Can you work these out from the model? Positions are in its coordinate system, mm. Face numbers are marked on the shaded views. A direction names the side the tool comes from. Round coordinates to 2 decimals unless told otherwise and drop trailing zeros. Loops run counter-clockwise (first coordinate to the right, second up) from the corner with the lowest first, then second, coordinate; pieces in that order, holes last. Notation, with made-up numbers: (13, 51.5) -> (54, 51.5) arc R30 ccw to (54, 79.5) -> close; hole circle Ø5 at (45, -1). An arc over 180 degrees is marked (long way). Use a Markdown table: item, result.
from build123d import *

# Parameters (mm, degrees)
BOSS_EXTRU_1_DEPTH = 75
SKETCH3_R          = 30
CUT_EXTRUDE3_DEPTH = 10
ESQUISSE2_R        = 45
BOSS_EXTRU_2_DEPTH = 8
CHANFREIN1_SIZE    = 5
BOSS_EXTRU_3_START = 8
ESQUISSE3_R        = 45
BOSS_EXTRU_3_DEPTH = 8
CHANFREIN2_SIZE    = 5
D_POUILLE5_ANGLE   = 45
D_POUILLE6_ANGLE   = 45
CHANFREIN4_SIZE    = 10
SKETCH2_R          = 45
CUT_EXTRUDE2_DEPTH = 55
FILLET1_R          = 5
CHAMFER1_SIZE      = 8


with BuildPart() as part:
    # Esquisse1 → Boss.-Extru.1 (new body)
    with BuildSketch(Plane.XY):
        with BuildLine():
            Line((95, -48), (95, 48))
            Line((95, 48), (-50, 48))
            Line((-50, 48), (-50, 42))
            Line((-50, 42), (-233.844505579, 42))
            ThreePointArc((-233.844505579, 42), (-295, 0), (-233.844505579, -42))
            Line((-233.844505579, -42), (-50, -42))
            Line((-50, -42), (-50, -48))
            Line((-50, -48), (95, -48))
        make_face()
    extrude(amount=BOSS_EXTRU_1_DEPTH)

    # Sketch3 → Cut-Extrude3 (cut)
    with BuildSketch(Plane.XY.offset(75)):
        Circle(SKETCH3_R)
    extrude(amount=-CUT_EXTRUDE3_DEPTH, mode=Mode.SUBTRACT)

    # Esquisse2 → Boss.-Extru.2 (add)
    with BuildSketch(Plane.XY.offset(75)):
        with Locations(Location((-250, 0, 0), (0, 0, 68.960530219))):
            Circle(ESQUISSE2_R)
    extrude(amount=BOSS_EXTRU_2_DEPTH)

    # Chanfrein1
    chanfrein1_edges = [part.edges().sort_by_distance(p)[0] for p in [
        (-266.155494421, -42, 83),
    ]]
    chamfer(chanfrein1_edges, length=CHANFREIN1_SIZE)

    # Esquisse3 → Boss.-Extru.3 (add)
    with BuildSketch(Plane(origin=(0, 0, 0), x_dir=(-1, 0, 0), z_dir=(0, 0, -1)).offset(BOSS_EXTRU_3_START)):
        with Locations((250, 0)):
            Circle(ESQUISSE3_R)
    extrude(amount=-BOSS_EXTRU_3_DEPTH)

    # Chanfrein2
    chanfrein2_edges = [part.edges().sort_by_distance(p)[0] for p in [
        (-205, 0, -8),
    ]]
    chamfer(chanfrein2_edges, length=CHANFREIN2_SIZE)

    # Dépouille5
    d_pouille5_faces = [part.faces().sort_by_distance(p)[0] for p in [
        (-50, 45, 37.5),
    ]]
    draft(d_pouille5_faces, Plane(origin=(-50, 42, 75), x_dir=(1, 0, 0), z_dir=(0, 1, 0)), D_POUILLE5_ANGLE)

    # Dépouille6
    d_pouille6_faces = [part.faces().sort_by_distance(p)[0] for p in [
        (-50, -45, 37.5),
    ]]
    draft(d_pouille6_faces, Plane(origin=(-50, -42, 75), x_dir=(-1, 0, 0), z_dir=(0, -1, 0)), D_POUILLE6_ANGLE)

    # Chanfrein4
    # the kernel refuses this chamfer: 10 mm, written as the material it takes off along each edge
    with BuildSketch(Plane(origin=(-259.561335458, -42, 75), x_dir=(0, -0.027495876610586317, -0.9996219169112968), z_dir=(1, 0, 0))) as chanfrein4_piece_1_section:
        Polygon((CHANFREIN4_SIZE * 0.999621916911, CHANFREIN4_SIZE * 0.0274958766106), (-CHANFREIN4_SIZE * 0.0274958766106, CHANFREIN4_SIZE * 0.999621916911), (0, 0), align=None)
    chanfrein4_piece_1 = extrude(amount=235.278165338, mode=Mode.PRIVATE)
    chanfrein4_piece_1 = chanfrein4_piece_1 - Plane(origin=(-250, 0, 71.650306889), x_dir=(0.35901098714230106, 0.9333333333333331, 0), z_dir=(0, 0, -1)) * Cylinder(45, 511, mode=Mode.PRIVATE)
    chanfrein4_piece_1 = split(chanfrein4_piece_1, bisect_by=Plane(origin=(-96.832103128, 4.832103128, 71.650306889), z_dir=(-0.7071067811865462, -0.7071067811865488, 0)), keep=Keep.TOP, mode=Mode.PRIVATE)
    add(chanfrein4_piece_1, mode=Mode.SUBTRACT)
    with BuildSketch(Plane(origin=(-259.561335458, -42, 0), x_dir=(0, 0.9996219169112968, -0.027495876610586372), z_dir=(1, 0, 0))) as chanfrein4_piece_2_section:
        Polygon((CHANFREIN4_SIZE * 0.999621916911, CHANFREIN4_SIZE * 0.0274958766106), (-CHANFREIN4_SIZE * 0.0274958766106, CHANFREIN4_SIZE * 0.999621916911), (0, 0), align=None)
    chanfrein4_piece_2 = extrude(amount=235.278165338, mode=Mode.PRIVATE)
    chanfrein4_piece_2 = chanfrein4_piece_2 - Plane(origin=(-250, 0, 3.349693111), x_dir=(-1, 0, 0), z_dir=(0, 0, -1)) * Cylinder(45, 511, mode=Mode.PRIVATE)
    chanfrein4_piece_2 = split(chanfrein4_piece_2, bisect_by=Plane(origin=(-96.832103062, 4.832103062, 3.349693111), z_dir=(-0.7071067811865462, -0.7071067811865488, 0)), keep=Keep.TOP, mode=Mode.PRIVATE)
    add(chanfrein4_piece_2, mode=Mode.SUBTRACT)
    with BuildSketch(Plane(origin=(-24.28317012, 42, 0), x_dir=(0, -0.9996219169112968, -0.027495876610586372), z_dir=(-1, 0, 0))) as chanfrein4_piece_3_section:
        Polygon((CHANFREIN4_SIZE * 0.999621916911, CHANFREIN4_SIZE * 0.0274958766106), (-CHANFREIN4_SIZE * 0.0274958766106, CHANFREIN4_SIZE * 0.999621916911), (0, 0), align=None)
    chanfrein4_piece_3 = extrude(amount=235.278165338, mode=Mode.PRIVATE)
    chanfrein4_piece_3 = chanfrein4_piece_3 - Plane(origin=(-250, 0, 3.349693112), x_dir=(-1, 0, 0), z_dir=(0, 0, -1)) * Cylinder(45, 511, mode=Mode.PRIVATE)
    chanfrein4_piece_3 = split(chanfrein4_piece_3, bisect_by=Plane(origin=(-96.832103108, -4.832103108, 3.349693112), z_dir=(-0.7071067811865462, 0.7071067811865488, 0)), keep=Keep.TOP, mode=Mode.PRIVATE)
    add(chanfrein4_piece_3, mode=Mode.SUBTRACT)
    with BuildSketch(Plane(origin=(-24.28317012, 42, 75), x_dir=(0, 0.027495876610586317, -0.9996219169112968), z_dir=(-1, 0, 0))) as chanfrein4_piece_4_section:
        Polygon((CHANFREIN4_SIZE * 0.999621916911, CHANFREIN4_SIZE * 0.0274958766106), (-CHANFREIN4_SIZE * 0.0274958766106, CHANFREIN4_SIZE * 0.999621916911), (0, 0), align=None)
    chanfrein4_piece_4 = extrude(amount=235.278165338, mode=Mode.PRIVATE)
    chanfrein4_piece_4 = chanfrein4_piece_4 - Plane(origin=(-250, 0, 71.65030689), x_dir=(0.35901098714230106, 0.9333333333333331, 0), z_dir=(0, 0, -1)) * Cylinder(45, 511, mode=Mode.PRIVATE)
    chanfrein4_piece_4 = split(chanfrein4_piece_4, bisect_by=Plane(origin=(-96.832103072, -4.832103072, 71.65030689), z_dir=(-0.7071067811865462, 0.7071067811865488, 0)), keep=Keep.TOP, mode=Mode.PRIVATE)
    add(chanfrein4_piece_4, mode=Mode.SUBTRACT)

    # Sketch2 → Cut-Extrude2 (cut)
    with BuildSketch(Plane(origin=(0, 0, 12), x_dir=(-1, 0, 0), z_dir=(0, 0, -1))):
        with Locations(Location((250, 0, 0), (0, 0, 242.733955549))):
            Circle(SKETCH2_R)
    extrude(amount=-CUT_EXTRUDE2_DEPTH, mode=Mode.SUBTRACT)

    # Fillet1
    # the kernel refuses this fillet: 5 mm, written as the material it takes off along each edge
    with BuildSketch(Plane(origin=(-233.844505579, -42, 12), x_dir=(0.8512324625883901, 0.5247888095564778, 0), z_dir=(0, 0, 1))) as fillet1_piece_1_section:
        with BuildLine():
            CenterArc((17.499102813, -4.914442902), FILLET1_R, 100.614557324, 137.73141557)
            Line((14.875158765, -9.170605214), (0, 0))
            ThreePointArc((0, 0), (8.289048701, -0.770013886), (16.578097401, 0))
        make_face()
    fillet1_piece_1 = extrude(amount=96.68712255, mode=Mode.PRIVATE)
    fillet1_piece_1 = split(fillet1_piece_1, bisect_by=Plane(origin=(-224.59334288, -39.762552666, 67), z_dir=(0, 0, -1)), keep=Keep.TOP, mode=Mode.PRIVATE)
    add(fillet1_piece_1, mode=Mode.SUBTRACT)
    with BuildSketch(Plane(origin=(-233.844505579, 42, 12), x_dir=(0.8512324625883905, -0.5247888095564773, 0), z_dir=(0, 0, 1))) as fillet1_piece_2_section:
        with BuildLine():
            CenterArc((17.499102813, 4.914442902), FILLET1_R, 121.654027105, 137.73141557)
            Line((14.875158765, 9.170605214), (0, 0))
            ThreePointArc((0, 0), (8.289048701, 0.770013886), (16.578097401, 0))
        make_face()
    fillet1_piece_2 = extrude(amount=96.68712255, mode=Mode.PRIVATE)
    fillet1_piece_2 = split(fillet1_piece_2, bisect_by=Plane(origin=(-224.59334288, 39.762552666, 67), z_dir=(0, 0, -1)), keep=Keep.TOP, mode=Mode.PRIVATE)
    add(fillet1_piece_2, mode=Mode.SUBTRACT)

    # Chamfer1
    chamfer1_edges = [part.edges().sort_by_distance(p)[0] for p in [
        (25.5, 48, 0),
        (95, 48, 37.5),
        (95, -48, 37.5),
        (25.5, -48, 75),
        (95, 0, 75),
        (25.5, 48, 75),
        (95, 0, 0),
        (25.5, -48, 0),
    ]]
    chamfer(chamfer1_edges, length=CHAMFER1_SIZE)


solid = part.part
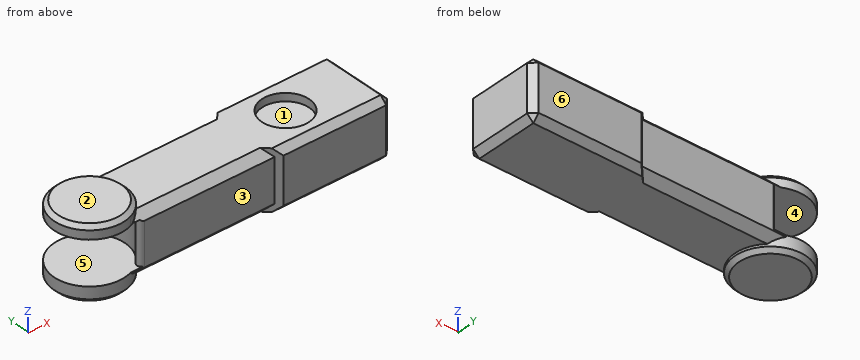
1. If we mould it in two halves opening along Y, with no side actions, what happens to the marked faces 1, 2, 3 and 4? For each: +Y half, -Y half, draft (parallel to the pull), parting line (faces both ways), or undercut.
Answer sheet:
| item | result |
|---|---|
| face 1 | undercut |
| face 2 | draft |
| face 3 | -Y half |
| face 4 | undercut |
2. I need wall thicknesses on line 1 (Z direction, x = -275, y = -14); line 2 (Y direction, x = 0, z = 67); line 3 (Y direction, x = -133, z = 51). Which ranges of each line are inside material? Lowest first, please.
Answer sheet:
| item | result |
|---|---|
| line 1 | z = -8 to 12, 67 to 83 |
| line 2 | y = -48 to -30, 30 to 48 |
| line 3 | y = -42 to 42 |
3. Which directions (+Z, -Z, +X, -X, +Y, -Y) give clear straight access to the entire face, cutting with the end or side of a thin tool? Please do the marked faces 5 and 6.
Answer sheet:
| item | result |
|---|---|
| face 5 | -X |
| face 6 | +Z, -Z, +X, -X, +Y |
4. I want a section at D-D (x = 43). Please give me the cut outline in (y, z).
Answer sheet:
| item | result |
|---|---|
| outline | (-48, 8) -> (-40, 0) -> (40, 0) -> (48, 8) -> (48, 67) -> (40, 75) -> (-40, 75) -> (-48, 67) -> close |
5. I want a section at B-B (y = 0). Please give me the cut outline in (x, z), plus the area to 3 significant figures.
Answer sheet:
| item | result |
|---|---|
| outline | (-295, -3) -> (-290, -8) -> (-210, -8) -> (-205, -3) -> (-205, 0) -> (87, 0) -> (95, 8) -> (95, 67) -> (87, 75) -> (30, 75) -> (30, 65) -> (-30, 65) -> (-30, 75) -> (-205, 75) -> (-205, 78) -> (-210, 83) -> (-290, 83) -> (-295, 78) -> (-295, 67) -> (-205, 67) -> (-205, 12) -> (-295, 12) -> close |
| area | 25,000 mm² |
6. Will these pins go through, and if not, where does the flat tip stop? pin 1 Ø6 at (x, y) = (5, -23) entering from -Z; pin 2 Ø10 at (x, y) = (-222, 29.5) entering from -Z; pin 3 Ø6 at (y, z) = (-30, 73) entering from +X; pin 4 Ø16.5 at (x, z) = (-104.5, 31.5) entering from +Y.
Answer sheet:
| item | result |
|---|---|
| pin 1 | stops at z = 0 |
| pin 2 | stops at z = -8 |
| pin 3 | stops at x = 92 |
| pin 4 | stops at y = 42 |
7. I want a section at A-A (x = -250). Please give me the cut outline in (y, z).
Answer sheet:
| item | result |
|---|---|
| outline | (-45, -3) -> (-40, -8) -> (40, -8) -> (45, -3) -> (45, 12) -> (-45, 12) -> close; (-45, 67) -> (45, 67) -> (45, 78) -> (40, 83) -> (-40, 83) -> (-45, 78) -> close |
8. I want a section at C-C (z = 42). Please give me the cut outline in (x, y), plus the area to 3 significant figures.
Answer sheet:
| item | result |
|---|---|
| outline | (-219.73, -33.3) arc R5 ccw to (-216.37, -42) -> (-50, -42) -> (-44, -48) -> (87, -48) -> (95, -40) -> (95, 40) -> (87, 48) -> (-44, 48) -> (-50, 42) -> (-216.37, 42) arc R5 ccw to (-219.73, 33.3) arc R45 cw to start |
| area | 27,400 mm² |
